Print and shaded views of the part. All mm, measured from the part's lowest x, y and z. A direction names the side the tool comes from. Round coordinates to 2 decimals unless told otherwise and drop trailing zeros. Order: outer loops, then holes, each group sorted by start corner. A loop starts at its lowest first (then second) coordinate and runs counter-clockwise, first axis right, second up. Notation, with made-up numbers: (19.5, 19.25) - (62.5, 19.25) arc R9 cw to (62.5, 28.25) - close; hole circle Ø3 at (-31, -14). An arc over 180 degrees is marked (long way). Write item = value, one per line. Start each with the question number.
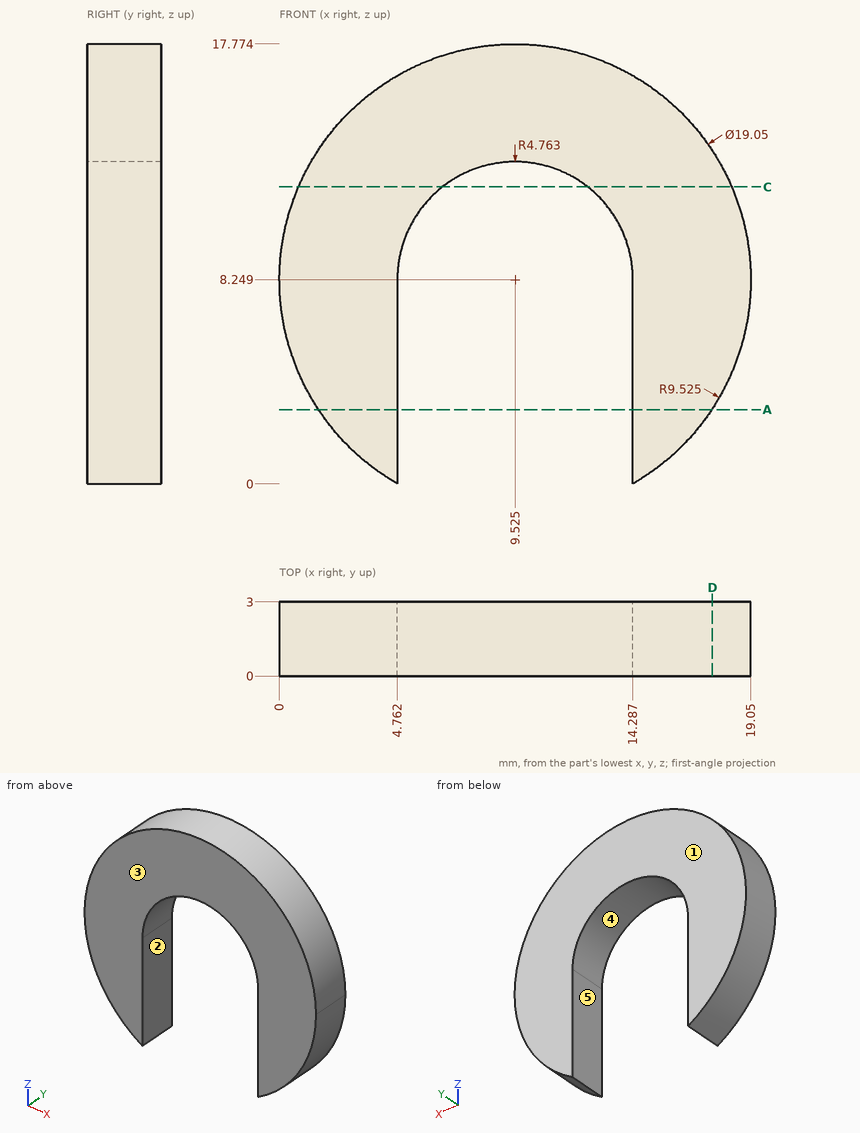
Item 1: Drop a flat-ended pin along its axis: pin 1 (0.9 mm diameter, centred on y = 2, z = 4.5, fed in from +X). Give the stop position or say it passes through.
Item 2: Saw through at D-D, the plane x = 17.5. Give the cut face in (y, z).
Item 3: Saw through at C-C, the plane z = 12. Give the cut face in (x, y).
Item 4: Probe L1, parallel to X at y = 1.25, z = 8.25; L2, parallel to X at y = 2.2, z = 1.25 (1 decimal); L3, parallel to Z at x = 9.5, y = 0.8. List the from-to ranges inside material, lowest first.
Item 5: Which spindle directions (+Z, -Z, +X, -X, +Y, -Y) get a long thin tool onto all of the face, cutting with end or side? Do the marked faces 1 and 2. Say none if no direction does.
Item 6: Mould opens along X. For the marked faces 3, 4 and 5 say: +X half, -X half, draft (parallel to the pull), parting line (faces both ways), or undercut.
Item 7: Saw through at A-A, the plane z = 3. Give the cut face in (x, y).
Check sheet entries:
q1.pin_1 = 18.46
q2.outline = (0, 3.04) - (3, 3.04) - (3, 13.46) - (0, 13.46) - close
q3.outline = (0.77, 0) - (6.59, 0) - (6.59, 3) - (0.77, 3) - close; (12.46, 0) - (18.28, 0) - (18.28, 3) - (12.46, 3) - close
q4.L1 = 0 to 4.76, 14.29 to 19.05
q4.L2 = 3.1 to 4.8, 14.3 to 16
q4.L3 = 13.01 to 17.77
q5.face_1 = +Z, -Z, +X, -X, +Y
q5.face_2 = -Z, +Y, -Y
q6.face_3 = draft
q6.face_4 = undercut
q6.face_5 = undercut
q7.outline = (1.58, 0) - (4.76, 0) - (4.76, 3) - (1.58, 3) - close; (14.29, 0) - (17.47, 0) - (17.47, 3) - (14.29, 3) - close
